Check sheet for the drawn part. Datum: minimum x, y, z corner. Units: mm. A direction names the side the tool comes from. Coordinates: 2 decimals unless noted, no trailing zeros. Loops run counter-clockwise (first coordinate to the right, second up) from the corner with the lowest first, then second, coordinate; pieces in that order, holes last.
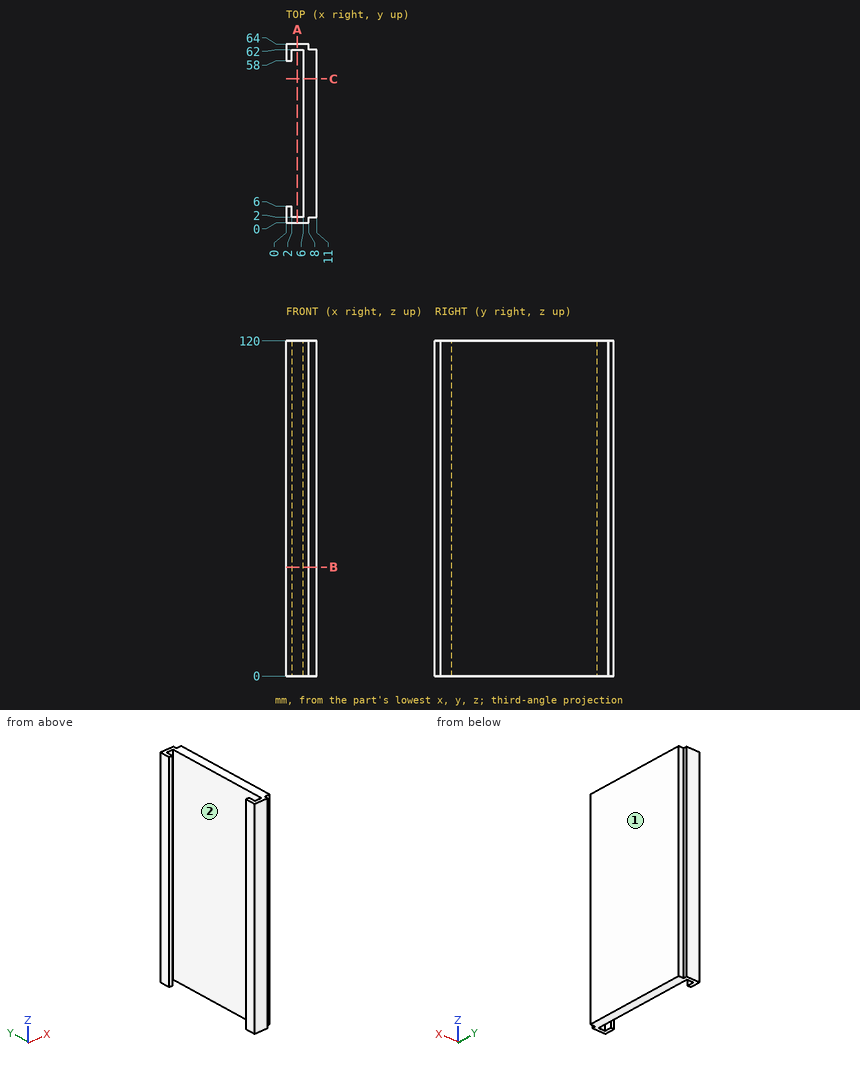
(1) Sectioned sample at A-A on x = 4. Record the cut outline in (y, z).
Findings:
outline: (0, 0) - (2, 0) - (2, 120) - (0, 120) - close; (62, 0) - (64, 0) - (64, 120) - (62, 120) - close
(2) Sectioned sample at B-B on z = 39. Record the cut outline in (x, y).
Findings:
outline: (0, 0) - (8, 0) - (8, 2) - (11, 2) - (11, 62) - (8, 62) - (8, 64) - (0, 64) - (0, 58) - (2, 58) - (2, 62) - (6, 62) - (6, 2) - (2, 2) - (2, 6) - (0, 6) - close
(3) Gauge pin test, flat ends, axial feed: pin 1 Ø1 at (x, z) = (0.5, 40.5) entering from -Y; pin 2 Ø2.5 at (x, z) = (9.5, 31.5) entering from +Y; pin 3 Ø1.6 at (y, z) = (63.5, 67.5) entering from +X; pin 4 Ø1.5 at (x, y) = (3.5, 9) entering from -Z. Record the tip position at first contact, or that the pin passes through.
Findings:
pin 1: stops at y = 0
pin 2: stops at y = 62
pin 3: stops at x = 8
pin 4: passes through
(4) Access from +Z, -Z, +X, -X, +Y, -Y to the whole of each face (thin tool, end or side, straight path). Record for the marked faces 1 and 2.
Findings:
face 1: +Z, -Z, +X, +Y, -Y
face 2: +Z, -Z
(5) Scan lines: L1, parallel to Y at x = 1, z = 37; L2, parallel to Y at x = 2.25, z = 69; L3, parallel to Y at x = 9.75, z = 32. Record each from-to range of solid material in increasing order.
Findings:
L1: y = 0 to 6, 58 to 64
L2: y = 0 to 2, 62 to 64
L3: y = 2 to 62
(6) Sectioned sample at C-C on y = 51.5. Record the cut outline in (x, z), and give its area (3 significant figures).
Findings:
outline: (6, 0) - (11, 0) - (11, 120) - (6, 120) - close
area: 600 mm2
